```python
from build123d import *

# Parameters (mm, degrees)
CROQUIS1_R              = 18.5
SALIENTE_EXTRUIR1_DEPTH = 18
CROQUIS2_R              = 16.5
SALIENTE_EXTRUIR2_DEPTH = 22.5
CROQUIS3_R              = 4.5
SALIENTE_EXTRUIR3_DEPTH = 3
CROQUIS4_R              = 1
SALIENTE_EXTRUIR4_DEPTH = 10.5
CROQUIS5_W              = 2.9
CROQUIS5_H              = 0.5
SALIENTE_EXTRUIR5_DEPTH = 6.3
CROQUIS6_R              = 6
SALIENTE_EXTRUIR6_DEPTH = 4.6
CROQUIS7_R              = 3
SALIENTE_EXTRUIR7_DEPTH = 6
SALIENTE_EXTRUIR8_DEPTH = 12
CROQUIS9_R              = 1.5
CORTAR_EXTRUIR1_DEPTH   = 5


with BuildPart() as part:
    # Croquis1 → Saliente-Extruir1 (new body)
    with BuildSketch(Plane.XY):
        Circle(CROQUIS1_R)
    extrude(amount=SALIENTE_EXTRUIR1_DEPTH)

    # Croquis2 → Saliente-Extruir2 (add)
    with BuildSketch(Plane.XY.offset(18)):
        Circle(CROQUIS2_R)
    extrude(amount=SALIENTE_EXTRUIR2_DEPTH)

    # Croquis3 → Saliente-Extruir3 (add)
    with BuildSketch(Plane.XY.offset(40.5)):
        Circle(CROQUIS3_R)
    extrude(amount=SALIENTE_EXTRUIR3_DEPTH)

    # Croquis4 → Saliente-Extruir4 (add)
    with BuildSketch(Plane.XY.offset(43.5)):
        Circle(CROQUIS4_R)
    extrude(amount=SALIENTE_EXTRUIR4_DEPTH)

    # Croquis5 → Saliente-Extruir5 (add)
    with BuildSketch(Plane.XY.offset(40.5)):
        with Locations((0, 12.25)):
            Rectangle(CROQUIS5_W, CROQUIS5_H)
        with Locations((0, -12.25)):
            Rectangle(CROQUIS5_W, CROQUIS5_H)
    extrude(amount=SALIENTE_EXTRUIR5_DEPTH)

    # Croquis6 → Saliente-Extruir6 (add)
    with BuildSketch(Plane(origin=(0, 0, 0), x_dir=(-1, 0, 0), z_dir=(0, 0, -1))):
        with Locations((0, -7)):
            Circle(CROQUIS6_R)
    extrude(amount=SALIENTE_EXTRUIR6_DEPTH)

    # Croquis7 → Saliente-Extruir7 (add)
    with BuildSketch(Plane(origin=(0, 0, -4.6), x_dir=(-1, 0, 0), z_dir=(0, 0, -1))):
        with Locations((0, -7)):
            Circle(CROQUIS7_R)
    extrude(amount=SALIENTE_EXTRUIR7_DEPTH)

    # Croquis8 → Saliente-Extruir8 (add)
    with BuildSketch(Plane(origin=(0, 0, -10.6), x_dir=(-1, 0, 0), z_dir=(0, 0, -1))):
        with BuildLine():
            Line((-1.658312395, -4.5), (1.658312395, -4.5))
            ThreePointArc((1.658312395, -4.5), (0, -10), (-1.658312395, -4.5))
        make_face()
    extrude(amount=SALIENTE_EXTRUIR8_DEPTH)

    # Croquis9 → Cortar-Extruir1 (cut)
    with BuildSketch(Plane(origin=(0, 0, 0), x_dir=(-1, 0, 0), z_dir=(0, 0, -1))):
        with Locations((-7.75, 13.423393759)):
            Circle(CROQUIS9_R)
        with Locations((-15.5, 0)):
            Circle(CROQUIS9_R)
        with Locations((-7.75, -13.423393759)):
            Circle(CROQUIS9_R)
        with Locations((15.5, 0)):
            Circle(CROQUIS9_R)
    extrude(amount=-CORTAR_EXTRUIR1_DEPTH, mode=Mode.SUBTRACT)


solid = part.part
```
Check sheet for the modelled part. Datum: model origin and axes. Units: mm. A direction names the side the tool comes from. Round coordinates to 2 decimals unless told otherwise and drop trailing zeros. Order: outer loops, then holes, each group sorted by start corner. A loop starts at its lowest first (then second) coordinate and runs counter-clockwise, first axis right, second up. Notation, with made-up numbers: M 77.25,17 L 135.25,17 A17 ccw 135.25,42 Z; hole C 23.25,-8.75 d4. An arc over 180 degrees is marked long. Answer in a Markdown table with one row per item.
(1) Draft check along X on faces 4 (the cylindrical face through (15.24, -6.32, 29.09)), 5 (the cylindrical face through (17, 0, 2)), 6 (the cylindrical face through (8.08, 11.96, 2.46)), 7 (the flat face through (0, 12, 44)). Enter one of: +X half, -X half, draft (parallel to the pull), parting line (faces both ways), or undercut.
Findings:
| item | result |
|---|---|
| face 4 | parting line |
| face 5 | undercut |
| face 6 | undercut |
| face 7 | draft |
(2) Material ranges on line 1 along Y through (x, z) = (0, 2.5); line 2 along Z through (x, y) = (6, 10.5); line 3 along Z through (x, y) = (-15.5, 0.5), recorded low to high. Write a range as from..to.
Findings:
| item | result |
|---|---|
| line 1 | y = -18.5..18.5 |
| line 2 | z = 0..40.5 |
| line 3 | z = 5..40.5 |
(3) Section check B-B on y = 6.5. Record the boundary of the cut face in (x, z).
Findings:
| item | result |
|---|---|
| outline | M -17.32,0 L 17.32,0 L 17.32,18 L 15.17,18 L 15.17,40.5 L -15.17,40.5 L -15.17,18 L -17.32,18 Z |
(4) Set-up check for faces 1 (the cylindrical face through (0, -1, 49)), 2 (the flat face through (0, -12.5, 44)), 3 (the flat face through (-15, 0, 5)): record each of +Z, -Z, +X, -X, +Y, -Y from which the full face is reachable in a straight line by a thin tool's end or side.
Findings:
| item | result |
|---|---|
| face 1 | +Z |
| face 2 | +Z, +X, -X, -Y |
| face 3 | -Z |
(5) Gauge pin test, flat ends, axial feed: pin 1 (5 mm diameter, centred on x = 10.5, y = -14, fed in from -Z); pin 2 (1.5 mm diameter, centred on x = 8, y = 13, fed in from -Z); pin 3 (5 mm diameter, centred on y = -1.5, z = 14, fed in from +X); pin 4 (0.6 mm diameter, centred on y = 12.5, z = 42.5, fed in from +X). Record the tip position at first contact, or that the pin passes through.
Findings:
| item | result |
|---|---|
| pin 1 | stops at z = 0 |
| pin 2 | stops at z = 5 |
| pin 3 | stops at x = 18.5 |
| pin 4 | stops at x = 1.45 |
(6) Section check C-C on z = 3.5. Record the boundary of the cut face in (x, y), plus the area to 3 significant figures.
Findings:
| item | result |
|---|---|
| outline | C 0,0 d37; hole C -15.5,0 d3; hole C 7.75,-13.42 d3; hole C 7.75,13.42 d3; hole C 15.5,0 d3 |
| area | 1,050 mm^2 |
(7) Section check D-D on z = 32. Record the boundary of the cut face in (x, y), plus the area to 3 significant figures.
Findings:
| item | result |
|---|---|
| outline | C 0,0 d33 |
| area | 855 mm^2 |
